Geometry: final body of the model. Coordinates: model frame, mm. A direction names the side the tool comes from. Give positions to 0.01 mm unless a question says otherwise; leave off trailing zeros. Write each loop counter-clockwise with the first axis right and the second up, starting at its lowest first coordinate (ties: lowest second). Pieces come first, ordered by that corner, then holes. Notation, with made-up numbers: (-35.75, 54.5) -> (-22.75, 54.5) arc R22 cw to (-22.75, 70.5) -> close; hole circle Ø8 at (28, 5.25). An arc over 180 degrees is marked (long way). Use CSV: the item, a comma, the result in double quotes. Start each with the question number.
1) Section C-C (z = 0). Count the separate pieces of the cut face and the enclosed holes in it, plus the area to 3 significant figures.
2) Section B-B (x = -10). Output: boundary loops of the cut face in (y, z), plus the area to 3 significant figures.
3) Material intervals for line 1 (Z direction, x = 8, y = -53); line 2 (Y direction, x = -15, z = -9.5); line 3 (Z direction, x = 6.5, y = 12), sorted ascending. Write a range as [from, to].
4) Set-up query: faces 1 (the face through (-20.3, 39.3, -9.45)), 2 (the face through (6, 36, -9.45)), 3 (the face through (7, -36, -9.45)). Return all of +Z, -Z, +X, -X, +Y, -Y with unobstructed straight access to the full face (end or side cutting, diameter ignored); none if empty.
5) Section A-A (y = 25). Output: boundary loops of the cut face in (x, z).
6) Contact query for flat-ended pins moving along their axis: P1, Ø12, axis at y = 64, z = -6.5, coming from the -X side; P2, Ø4, axis at x = 3.5, y = 1.5, coming from the -Z side; P3, Ø1.1, axis at x = -13, z = -11, coming from the +Y side. Output: stop coordinate, or through.
7) Draft query along Z for faces 4 (the face through (-40, 36, -11)), 5 (the face through (6.9, 61.01, 6.45)), 6 (the face through (-13, 36, -13.2)), 7 (the face through (6.9, 103.95, -0.64)). Return one class per face: pulls with the +Z half, pulls with the -Z half, needs draft (parallel to the pull), parting line crosses it, or undercut.
```python
from build123d import *

# Parameters (mm, degrees)
SKETCH_1_R      = 4.95
EXTRUDE_1_DEPTH = 14
SKETCH_3_W      = 14
SKETCH_3_H      = 60.948164725
EXTRUDE_2_DEPTH = 3
SKETCH_4_R      = 4.95
EXTRUDE_3_DEPTH = 14
SKETCH_5_W      = 49
SKETCH_5_H      = 5.67
EXTRUDE_4_DEPTH = 1.75
EXTRUDE_5_DEPTH = 2


with BuildPart() as part:
    # Эскиз1 → Бобышка-Вытянуть1 (new body)
    with BuildSketch(Plane(origin=(0, 0, 0), x_dir=(0, 0, -1), z_dir=(1, 0, 0))):
        with BuildLine():
            Line((6.45, 38.092602953), (6.45, 53.329644134))
            ThreePointArc((6.45, 53.329644134), (0, 59.779644134), (-6.45, 53.329644134))
            Line((-6.45, 53.329644134), (-6.45, 38.092602953))
            Line((-6.45, 38.092602953), (-6.45, 22.855561772))
            Line((-6.45, 22.855561772), (-6.45, 7.618520591))
            Line((-6.45, 7.618520591), (-6.45, -7.618520591))
            ThreePointArc((-6.45, -7.618520591), (0, -14.068520591), (6.45, -7.618520591))
            Line((6.45, -7.618520591), (6.45, 7.618520591))
            Line((6.45, 7.618520591), (6.45, 22.855561772))
            Line((6.45, 22.855561772), (6.45, 38.092602953))
        make_face()
        with Locations((0, 7.618520591)):
            Circle(SKETCH_1_R, mode=Mode.SUBTRACT)
        with Locations((0, -7.618520591)):
            Circle(SKETCH_1_R, mode=Mode.SUBTRACT)
        with Locations((0, 22.855561772)):
            Circle(SKETCH_1_R, mode=Mode.SUBTRACT)
        with Locations((0, 38.092602953)):
            Circle(SKETCH_1_R, mode=Mode.SUBTRACT)
        with Locations((0, 53.329644134)):
            Circle(SKETCH_1_R, mode=Mode.SUBTRACT)
    extrude(amount=EXTRUDE_1_DEPTH)

    # Эскиз3 → Бобышка-Вытянуть2 (add)
    with BuildSketch(Plane(origin=(0, 0, -6.45), x_dir=(-1, 0, 0), z_dir=(0, 0, -1))):
        with Locations((-7, 22.855561772)):
            Rectangle(SKETCH_3_W, SKETCH_3_H)
    extrude(amount=EXTRUDE_2_DEPTH)

    # Эскиз4 → Бобышка-Вытянуть3 (add)
    with BuildSketch(Plane.ZY):
        with BuildLine():
            Line((-9.45, 53.329644134), (-9.45, 57.948164724))
            ThreePointArc((-9.45, 57.948164724), (-6.45, 60.948164724), (-9.45, 63.948164724))
            Line((-9.45, 63.948164724), (-9.45, 99.040767677))
            ThreePointArc((-9.45, 99.040767677), (0, 108.490767677), (9.45, 99.040767677))
            Line((9.45, 99.040767677), (9.45, 63.948164724))
            ThreePointArc((9.45, 63.948164724), (6.45, 60.948164724), (9.45, 57.948164724))
            Line((9.45, 57.948164724), (9.45, -12.237041181))
            ThreePointArc((9.45, -12.237041181), (6.45, -15.237041181), (9.45, -18.237041181))
            Line((9.45, -18.237041181), (9.45, -53.329644134))
            ThreePointArc((9.45, -53.329644134), (0, -62.779644134), (-9.45, -53.329644134))
            Line((-9.45, -53.329644134), (-9.45, -18.237041181))
            ThreePointArc((-9.45, -18.237041181), (-6.45, -15.237041181), (-9.45, -12.237041181))
            Line((-9.45, -12.237041181), (-9.45, 53.329644134))
        make_face()
        with Locations((0, 99.040767677)):
            Circle(SKETCH_4_R, mode=Mode.SUBTRACT)
        with Locations((0, 83.803726496)):
            Circle(SKETCH_4_R, mode=Mode.SUBTRACT)
        with Locations((0, 68.566685315)):
            Circle(SKETCH_4_R, mode=Mode.SUBTRACT)
        with Locations(Location((0, 53.329644134, 0), (0, 0, 180))):
            Circle(SKETCH_4_R, mode=Mode.SUBTRACT)
        with Locations((0, -53.329644134)):
            Circle(SKETCH_4_R, mode=Mode.SUBTRACT)
        with Locations((0, -38.092602953)):
            Circle(SKETCH_4_R, mode=Mode.SUBTRACT)
        with Locations((0, -22.855561772)):
            Circle(SKETCH_4_R, mode=Mode.SUBTRACT)
        with Locations(Location((0, -7.618520591, 0), (0, 0, 180))):
            Circle(SKETCH_4_R, mode=Mode.SUBTRACT)
        with Locations(Location((0, 38.092602953, 0), (0, 0, 180))):
            Circle(SKETCH_4_R, mode=Mode.SUBTRACT)
        with Locations(Location((0, 22.855561772, 0), (0, 0, 180))):
            Circle(SKETCH_4_R, mode=Mode.SUBTRACT)
        with Locations(Location((0, 7.618520591, 0), (0, 0, 180))):
            Circle(SKETCH_4_R, mode=Mode.SUBTRACT)
    extrude(amount=-EXTRUDE_3_DEPTH)

    # Эскиз5 → Бобышка-Вытянуть4 (add)
    with BuildSketch(Plane(origin=(0, 0, -9.45), x_dir=(-1, 0, 0), z_dir=(0, 0, -1))):
        Polygon((-14, 31.185355866), (-14, 40.855355866), (39, 40.855355866), (40, 40.855355866), (40, 31.185355866), (39, 31.185355866), align=None)
        with Locations((12.5, 36.020355866)):
            Rectangle(SKETCH_5_W, SKETCH_5_H, mode=Mode.SUBTRACT)
    extrude(amount=EXTRUDE_4_DEPTH)

    # Эскиз6 → Бобышка-Вытянуть5 (add)
    with BuildSketch(Plane(origin=(0, 0, -11.2), x_dir=(-1, 0, 0), z_dir=(0, 0, -1))):
        Polygon((39, 31.185355866), (-14, 31.185355866), (-14, 40.855355866), (39, 40.855355866), (40, 40.855355866), (40, 31.185355866), align=None)
    extrude(amount=EXTRUDE_5_DEPTH)


solid = part.part
```
Answers follow:
1,separate pieces,"12"
1,enclosed holes,"0"
1,area,"873 mm^2"
2,outline,"(31.19, -13.2) -> (40.86, -13.2) -> (40.86, -9.45) -> (38.86, -9.45) -> (38.86, -11.2) -> (33.19, -11.2) -> (33.19, -9.45) -> (31.19, -9.45) -> close"
2,area,"26.3 mm^2"
3,line 1,"z = [-9.45, -4.94], [4.94, 9.45]"
3,line 2,"y = [31.19, 33.19], [38.86, 40.86]"
3,line 3,"z = [-9.45, -2.3], [2.3, 9.45]"
4,face 1,"+Z, -X, +Y, -Y"
4,face 2,"none"
4,face 3,"-Z, +X, -X, -Y"
5,outline,"(0, -9.45) -> (14, -9.45) -> (14, -4.46) -> (0, -4.46) -> close; (0, 4.46) -> (14, 4.46) -> (14, 9.45) -> (0, 9.45) -> close"
6,P1,"stops at x = 0"
6,P2,"stops at z = -9.45"
6,P3,"stops at y = 40.86"
7,face 4,"needs draft"
7,face 5,"pulls with the +Z half"
7,face 6,"pulls with the -Z half"
7,face 7,"undercut"
